from build123d import *

# Parameters (mm, degrees)
SKETCH1_R                       = 12.7
BOSS_EXTRUDE1_DEPTH             = 317.5
SKETCH2_W                       = 393.7
SKETCH2_H                       = 622.3
CUT_EXTRUDE1_DEPTH              = 152.447724951
BOSS_EXTRUDE2_REACH             = 319.5
SKETCH3_R                       = 12.7
BOSS_EXTRUDE2_DIRECTION_2_REACH = 319.5


with BuildPart() as part:
    # Sketch1 → Boss-Extrude1 (new body, symmetric)
    with BuildSketch(Plane.XY):
        with BuildLine():
            Line((0, 0), (166.121717342, 0))
            ThreePointArc((166.121717342, 0), (170.203418664, -1.485617786), (172.375246574, -5.247334072))
            Line((172.375246574, -5.247334072), (182.331323933, -61.711054592))
            ThreePointArc((182.331323933, -61.711054592), (201.969223554, -85.741108229), (232.718040732, -81.545774931))
            Line((232.718040732, -81.545774931), (349.319070642, 6.40195002))
            ThreePointArc((349.319070642, 6.40195002), (360.307001568, 41.83121801), (330.2, 63.5))
            Line((330.2, 63.5), (0, 63.5))
            ThreePointArc((0, 63.5), (-31.75, 31.75), (0, 0))
        make_face()
        with Locations((0, 31.75)):
            Circle(SKETCH1_R, mode=Mode.SUBTRACT)
    extrude(amount=BOSS_EXTRUDE1_DEPTH, both=True)

    # Sketch2 → Cut-Extrude1 (cut, through all)
    with BuildSketch(Plane(origin=(0, 63.5, 0), x_dir=(1, 0, 0), z_dir=(0, 1, 0))):
        with Locations((165.1, 0)):
            Rectangle(SKETCH2_W, SKETCH2_H)
    extrude(amount=-CUT_EXTRUDE1_DEPTH, mode=Mode.SUBTRACT)

    # Sketch3 → Boss-Extrude2 (add, up to next)
    with BuildSketch(Plane.XY, mode=Mode.PRIVATE) as boss_extrude2_sk1:
        with Locations((330.2, 31.75)):
            Circle(SKETCH3_R)
    boss_extrude2_tool1 = extrude(boss_extrude2_sk1.sketch, amount=BOSS_EXTRUDE2_REACH, mode=Mode.PRIVATE) - part.part
    add(boss_extrude2_tool1.solids().sort_by_distance((330.2, 31.75, 0))[0])
    # Sketch3 → Boss-Extrude2 (add, up to next)
    with BuildSketch(Plane.XY, mode=Mode.PRIVATE) as boss_extrude2_sk2:
        with Locations((213.598970091, -56.197724951)):
            Circle(SKETCH3_R)
    boss_extrude2_tool2 = extrude(boss_extrude2_sk2.sketch, amount=BOSS_EXTRUDE2_REACH, mode=Mode.PRIVATE) - part.part
    add(boss_extrude2_tool2.solids().sort_by_distance((213.59897, -56.197725, 0))[0])

    # Sketch3 → Boss-Extrude2 direction 2 (add, up to next)
    with BuildSketch(Plane.XY, mode=Mode.PRIVATE) as boss_extrude2_direction_2_sk1:
        with Locations((330.2, 31.75)):
            Circle(SKETCH3_R)
    boss_extrude2_direction_2_tool1 = extrude(boss_extrude2_direction_2_sk1.sketch, amount=-BOSS_EXTRUDE2_DIRECTION_2_REACH, mode=Mode.PRIVATE) - part.part
    add(boss_extrude2_direction_2_tool1.solids().sort_by_distance((330.2, 31.75, 0))[0])
    # Sketch3 → Boss-Extrude2 direction 2 (add, up to next)
    with BuildSketch(Plane.XY, mode=Mode.PRIVATE) as boss_extrude2_direction_2_sk2:
        with Locations((213.598970091, -56.197724951)):
            Circle(SKETCH3_R)
    boss_extrude2_direction_2_tool2 = extrude(boss_extrude2_direction_2_sk2.sketch, amount=-BOSS_EXTRUDE2_DIRECTION_2_REACH, mode=Mode.PRIVATE) - part.part
    add(boss_extrude2_direction_2_tool2.solids().sort_by_distance((213.59897, -56.197725, 0))[0])


solid = part.part
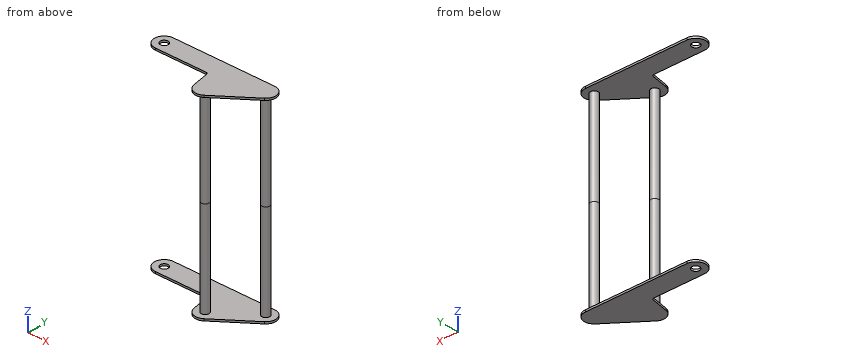
Check sheet for the modelled part. Datum: model origin and axes. Units: mm. Coordinates: 2 decimals unless noted, no trailing zeros. Write each loop counter-clockwise with the first axis right and the second up, starting at its lowest first coordinate (ties: lowest second). Pieces come first, ordered by that corner, then holes.
Item 1: Cross-section at B-B on x = 189. Record the boundary of the cut face in (y, z), then the cut area to 3 significant figures.
Numbers:
outline: (-76.27, -317.5) - (63.5, -317.5) - (63.5, -311.15) - (-76.27, -311.15) - close; (-76.27, 311.15) - (63.5, 311.15) - (63.5, 317.5) - (-76.27, 317.5) - close
area: 1,780 mm2
Item 2: Scan lines: probe 1 along Z at (x, y) = (261, 30); probe 2 along Y at (x, z) = (0, -313); probe 3 along X at (y, z) = (31.75, 313). Record each from-to range of solid material in increasing order.
Numbers:
probe 1: z = -317.5 to -311.15, 311.15 to 317.5
probe 2: y = 0 to 19.05, 44.45 to 63.5
probe 3: x = -31.75 to -12.7, 12.7 to 361.95
Item 3: Cross-section at C-C on z = 38.5. Record the boundary of the cut face in (x, y).
Numbers:
outline: circle Ø25.4 at (213.6, -56.2); circle Ø25.4 at (330.2, 31.75)
Item 4: Cross-section at A-A on y = 31.75. Record the boundary of the cut face in (x, z), then the cut area to 3 significant figures.
Numbers:
outline: (-31.75, -317.5) - (-12.7, -317.5) - (-12.7, -311.15) - (-31.75, -311.15) - close; (-31.75, 311.15) - (-12.7, 311.15) - (-12.7, 317.5) - (-31.75, 317.5) - close; (12.7, -317.5) - (361.95, -317.5) - (361.95, -311.15) - (342.9, -311.15) - (342.9, 311.15) - (361.95, 311.15) - (361.95, 317.5) - (12.7, 317.5) - (12.7, 311.15) - (317.5, 311.15) - (317.5, -311.15) - (12.7, -311.15) - close
area: 20,500 mm2
Item 5: Depth check by flat-ended pin: pin 1 Ø23 at (x, y) = (0, 31.75) entering from +Z; pin 2 Ø1 at (y, z) = (36.5, -21) entering from +X; pin 3 Ø6 at (y, z) = (-43, -96.5) entering from -X; pin 4 Ø1.9 at (x, z) = (110, -315.5) entering from -Y. Enter the tip coordinate at first touch or a pass-through.
Numbers:
pin 1: passes through
pin 2: stops at x = 342.17
pin 3: stops at x = 206.03
pin 4: stops at y = 0
